Input: part model. Units: mm. Frame: model coordinates. A direction names the side the tool comes from. Give positions to 0.01 mm unless a question says otherwise; leave off trailing zeros. Loops run counter-clockwise (first coordinate to the right, second up) from the corner with the lowest first, then second, coordinate; pieces in that order, holes last.
from build123d import *

# Parameters (mm, degrees)
SKETCH_1_W          = 50
SKETCH_1_H          = 29.7
EXTRUDE_1_DEPTH     = 2
SKETCH_2_W          = 50
SKETCH_2_H          = 29.7
SKETCH_2_W_2        = 46
SKETCH_2_H_2        = 25.7
EXTRUDE_2_DEPTH     = 26
SKETCH_4_R          = 1.5
CUT_EXTRUDE_2_DEPTH = 2
SKETCH_5_R          = 1.5
CUT_EXTRUDE_3_DEPTH = 2
SKETCH_3_R          = 1
CUT_EXTRUDE_5_DEPTH = 2


with BuildPart() as part:
    # 草图1 → 凸台-拉伸1 (new body)
    with BuildSketch(Plane(origin=(0, 0, 0), x_dir=(1, 0, 0), z_dir=(0, 1, 0))):
        Rectangle(SKETCH_1_W, SKETCH_1_H)
    extrude(amount=EXTRUDE_1_DEPTH)

    # 草图2 → 凸台-拉伸2 (add)
    with BuildSketch(Plane(origin=(0, 2, 0), x_dir=(1, 0, 0), z_dir=(0, 1, 0))):
        Rectangle(SKETCH_2_W, SKETCH_2_H)
        Rectangle(SKETCH_2_W_2, SKETCH_2_H_2, mode=Mode.SUBTRACT)
    extrude(amount=EXTRUDE_2_DEPTH)

    # 草图4 → 切除-拉伸2 (cut)
    with BuildSketch(Plane(origin=(25, 0, 0), x_dir=(0, 0, -1), z_dir=(1, 0, 0))):
        with Locations((-7.5, 12.1)):
            Circle(SKETCH_4_R)
        with Locations((-7.5, 22.1)):
            Circle(SKETCH_4_R)
        with Locations(Location((7.5, 12.1, 0), (0, 0, 180))):
            Circle(SKETCH_4_R)
        with Locations(Location((7.5, 22.1, 0), (0, 0, 180))):
            Circle(SKETCH_4_R)
        with BuildLine():
            ThreePointArc((-7.5, 18.1), (-4.671572875, 19.271572875), (-3.5, 22.1))
            ThreePointArc((-3.5, 22.1), (0, 25.6), (3.5, 22.1))
            ThreePointArc((3.5, 22.1), (4.671572875, 19.271572875), (7.5, 18.1))
            ThreePointArc((7.5, 18.1), (8.135409658, 17.1), (7.5, 16.1))
            ThreePointArc((7.5, 16.1), (4.671572875, 14.928427125), (3.5, 12.1))
            ThreePointArc((3.5, 12.1), (0, 8.6), (-3.5, 12.1))
            ThreePointArc((-3.5, 12.1), (-4.671572875, 14.928427125), (-7.5, 16.1))
            ThreePointArc((-7.5, 16.1), (-8.135409658, 17.1), (-7.5, 18.1))
        make_face()
    cut_extrude_2 = extrude(amount=-CUT_EXTRUDE_2_DEPTH, mode=Mode.SUBTRACT)

    # 镜向2: 切除-拉伸2 across plane
    add(cut_extrude_2.mirror(Plane(origin=(0, 0, 0), x_dir=(0, 0, 1), z_dir=(1, 0, 0))), mode=Mode.SUBTRACT)

    # 草图5 → 切除-拉伸3 (cut)
    with BuildSketch(Plane.XZ):
        with Locations(Location((7.5, 5, 0), (0, 0, 270))):
            Circle(SKETCH_5_R)
        with Locations(Location((7.5, -5, 0), (0, 0, 90))):
            Circle(SKETCH_5_R)
        with Locations(Location((-7.5, -5, 0), (0, 0, 270))):
            Circle(SKETCH_5_R)
        with Locations(Location((-7.5, 5, 0), (0, 0, 90))):
            Circle(SKETCH_5_R)
        with BuildLine():
            Line((7.5, 2.033504468), (13.445752083, 2.033504468))
            ThreePointArc((13.445752083, 2.033504468), (14.861299313, 1.433919229), (15.415512326, 0))
            ThreePointArc((15.415512326, 0), (14.861299313, -1.433919229), (13.445752083, -2.033504468))
            Line((13.445752083, -2.033504468), (7.5, -2.033504468))
            add(Edge.make_bspline(
                [(0, -7.23012785), (3.34126485, -7.578100632), (3.029788905, -1.842013201), (7.5, -2.033504468)],
                knots=[0, 0, 0, 0, 1, 1, 1, 1], degree=3))
            add(Edge.make_bspline(
                [(0, -7.23012785), (-3.34126485, -7.578100632), (-3.029788905, -1.842013201), (-7.5, -2.033504468)],
                knots=[0, 0, 0, 0, 1, 1, 1, 1], degree=3))
            Line((-7.5, -2.033504468), (-13.445752083, -2.033504468))
            ThreePointArc((-13.445752083, -2.033504468), (-14.861299313, -1.433919229), (-15.415512326, 0))
            ThreePointArc((-15.415512326, 0), (-14.861299313, 1.433919229), (-13.445752083, 2.033504468))
            Line((-13.445752083, 2.033504468), (-7.5, 2.033504468))
            add(Edge.make_bspline(
                [(0, 7.23012785), (-3.34126485, 7.578100632), (-3.029788905, 1.842013201), (-7.5, 2.033504468)],
                knots=[0, 0, 0, 0, 1, 1, 1, 1], degree=3))
            add(Edge.make_bspline(
                [(0, 7.23012785), (3.34126485, 7.578100632), (3.029788905, 1.842013201), (7.5, 2.033504468)],
                knots=[0, 0, 0, 0, 1, 1, 1, 1], degree=3))
        make_face()
    extrude(amount=-CUT_EXTRUDE_3_DEPTH, mode=Mode.SUBTRACT)

    # 草图3 → 切除-拉伸5 (cut)
    with BuildSketch(Plane.XY.offset(14.85)):
        with BuildLine():
            ThreePointArc((-20.1, 10.4), (-18.402943725, 9.697056275), (-17.7, 8))
            Line((-17.7, 8), (17.7, 8))
            ThreePointArc((17.7, 8), (18.402943725, 9.697056275), (20.1, 10.4))
            Line((20.1, 10.4), (20.1, 23.8))
            ThreePointArc((20.1, 23.8), (17.855005568, 25.351471863), (18.512549213, 28))
            Line((18.512549213, 28), (-18.512549213, 28))
            ThreePointArc((-18.512549213, 28), (-17.855005568, 25.351471863), (-20.1, 23.8))
            Line((-20.1, 23.8), (-20.1, 10.4))
        make_face()
        with Locations((-20.1, 8)):
            Circle(SKETCH_3_R)
        with Locations((20.1, 8)):
            Circle(SKETCH_3_R)
        with Locations((20.1, 26.2)):
            Circle(SKETCH_3_R)
        with Locations((-20.1, 26.2)):
            Circle(SKETCH_3_R)
    cut_extrude_5 = extrude(amount=-CUT_EXTRUDE_5_DEPTH, mode=Mode.SUBTRACT)

    # 镜向4: 切除-拉伸5 across plane
    add(cut_extrude_5.mirror(Plane.XY), mode=Mode.SUBTRACT)


solid = part.part
(1) Cut plane D-D (z = 1). Return the cut outline in (x, y), and give its area (3 significant figures).
Values follow:
outline: (-25, 0) - (-15.18, 0) - (-15.18, 2) - (-23, 2) - (-23, 8.75) - (-25, 8.75) - close; (-25, 25.45) - (-23, 25.45) - (-23, 28) - (-25, 28) - close; (15.18, 0) - (25, 0) - (25, 8.75) - (23, 8.75) - (23, 2) - (15.18, 2) - close; (23, 25.45) - (25, 25.45) - (25, 28) - (23, 28) - close
area: 76.4 mm2
(2) Cut plane C-C (y = 3). Return the cut outline in (x, z), and give its area (3 significant figures).
Values follow:
outline: (-25, -14.85) - (25, -14.85) - (25, 14.85) - (-25, 14.85) - close; hole (-23, -12.85) - (23, -12.85) - (23, 12.85) - (-23, 12.85) - close
area: 303 mm2
(3) Cut plane A-A (y = 26.2). Count the separate pieces of the cut face and the enclosed holes in it, and give its area (3 significant figures).
Values follow:
separate pieces: 6
enclosed holes: 0
area: 145 mm2
(4) Cut plane B-B (z = 11.75). Return the cut outline in (x, y).
Values follow:
outline: (-25, 0) - (25, 0) - (25, 28) - (23, 28) - (23, 2) - (-23, 2) - (-23, 28) - (-25, 28) - close
(5) Mould query, pull axis Y, two halves, no side actions, for faces 4 (the cylindrical face through (6, 1, 5)), 5 (the cylindrical face through (24.014, 19.303, -4.641)). Classes: +Y half, -Y half, draft (parallel to the pull), parting line (faces both ways), or undercut.
Values follow:
face 4: draft
face 5: undercut
(6) Ray query, probe 1 along Y at (x, z) = (24.3, -7.5); probe 2 along X at (y, z) = (11.75, 11.5); probe 3 along Z at (x, y) = (3.5, 6.75). Return the intervals inside material, ascending.
Values follow:
probe 1: y = 0 to 10.6, 13.6 to 16.1, 18.1 to 20.6, 23.6 to 28
probe 2: x = -25 to -23, 23 to 25
probe 3: z = -14.85 to -12.85, 12.85 to 14.85
(7) Reachability of faces 1 (the cylindrical face through (24.014, 19.241, 4.703)), 2 (the cylindrical face through (17.87, 25.31, 13.86)), 3 (the flat face through (-10, 1, -2.034)) from +Z, -Z, +X, -X, +Y, -Y: full face, straight path, thin tool, end or side. Return the list, or none.
Values follow:
face 1: +X, -X
face 2: +Z, -Z
face 3: +Y, -Y
(8) Pin query (flat end, axial travel): pin 1 Ø7.5 at (x, z) = (-4, 0.5) entering from +Y; pin 2 Ø2.5 at (x, y) = (20.1, 8) entering from +Z. Return the tip coordinate at first contact, or that it passes through.
Values follow:
pin 1: stops at y = 2
pin 2: stops at z = 14.85
